Build history of the part. All positions in model axes, mm. Face numbers are marked on the shaded views. A direction names the side the tool comes from. Give positions to 0.01 mm unless a question says otherwise; leave off trailing zeros. Order: outer loops, then holes, each group sorted by start corner. A loop starts at its lowest first (then second) coordinate and runs counter-clockwise, first axis right, second up. Notation, with made-up numbers: M -8.5,77 L 15.5,77 A9 cw 15.5,93 Z; hole C 34.25,37.25 d7. An arc over 180 degrees is marked long. Use CSV: the item, a comma, the result in double quotes. Start each with the question number.
Item 1: Band-saw the part on A-A on y = 47.5. Write the cut outline in (x, z).
Item 2: Band-saw the part on B-B on z = 26. Write the cut outline in (x, y), plus the area to 3 significant figures.
Item 3: Wall check: line 1 along X through (y, z) = (41, 72); line 2 along Y through (x, z) = (24.5, 47.5); line 3 along X through (y, z) = (38, 25). Give the ranges that are in metal, low to high.
Item 4: Which spindle directions (+Z, -Z, +X, -X, +Y, -Y) get a long thin tool onto all of the face, cutting with end or side? Do the marked faces 1 and 2. Say none if no direction does.
Item 5: Band-saw the part on D-D on z = 61. Write the cut outline in (x, y), plus the area to 3 significant figures.
Item 6: Band-saw the part on C-C on x = 17.5. Write the cut outline in (y, z).
Item 7: Two-plate mould, pull along Z, no slides. Class the marked faces 3, 4 and 5: pulls with the +Z half, pulls with the -Z half, needs draft (parallel to the pull), parting line crosses it, or undercut.
Item 8: Pin check, flat tips, straight feed: P1, Ø13, axis at y = 42, z = 54.5, coming from the +X side; P2, Ø6, axis at y = 25, z = 65.5, coming from the +X side; P3, Ø8, axis at y = 18.5, z = 9.5, coming from the +X side; P4, Ø4, axis at x = -39.5, y = 34, coming from the -Z side. Stop position of each tip, or through.
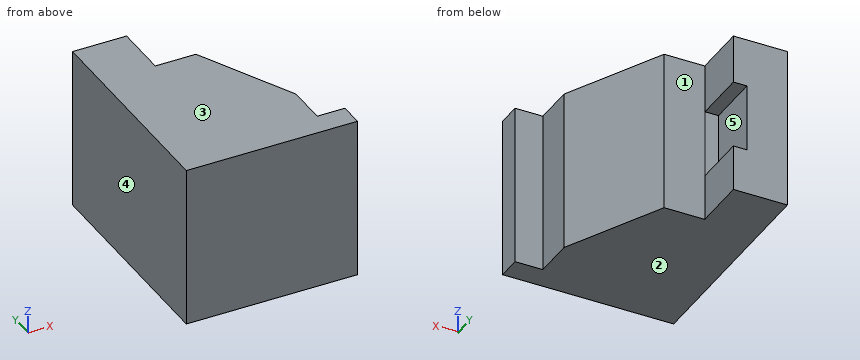
from build123d import *

# Parameters (mm, degrees)
F0_W      = 89.0809036791
F0_H      = 101.640611887
F1_DEPTH  = 76.2
F3_DEPTH  = 76.201
F4_R      = 10.6888946351
F3_FACE_W = 51.3844064591
F3_FACE_H = 76.2
F5_DEPTH  = 12.7
F8_W      = 6.35
F8_H      = 31.75
F9_DEPTH  = 25.4


# Not quite as in the source:
# - a feature of the source that left no trace in its solid (it failed there, or was rolled back) is left out


with BuildPart() as f1:
    # F0 (on Top) → F1 (new body)
    with BuildSketch(Plane.XY):
        with Locations((-6.628734991, 2.674754709)):
            Rectangle(F0_W, F0_H)
    extrude(amount=F1_DEPTH)

    # F2 (on face) → F3 (cut, through all)
    with BuildSketch(Plane.XY.offset(76.2)):
        Polygon((37.9117168486, 53.4950606525), (-25.8171800524, 53.4950606525), (-25.8171800524, 27.9104653746), (-6.7450297065, 27.9104653746), (16.0485189408, -18.1418024004), (16.0485189408, -36.9813665748), (29.0734022856, -36.9813665748), (29.0734022856, -48.1455512345), (31.1666838825, -48.1455512345), (37.9117168486, -48.1455512345), align=None)
    extrude(amount=-F3_DEPTH, mode=Mode.SUBTRACT)

    # F4 (on Right) + F3_face (on face) → F5 (join)
    with BuildSketch(Plane.YZ):
        with Locations((0, 59.542324394)):
            Circle(F4_R)
    with BuildSketch(Plane(origin=(4.6517446171, 4.8843314871, 38.1), x_dir=(-0.4435888282, 0.8962304121, 0), z_dir=(0.8962304121, 0.4435888282, 0))):
        Rectangle(F3_FACE_W, F3_FACE_H)
    extrude(amount=-F5_DEPTH, dir=(1, 0, 0))

    # F8 (on face) → F9 (cut)
    with BuildSketch(Plane(origin=(0, 53.4950606525, 0), x_dir=(-1, 0, 0), z_dir=(0, 1, 0))):
        with Locations((28.9921800524, 37.465)):
            Rectangle(F8_W, F8_H)
    extrude(amount=-F9_DEPTH, mode=Mode.SUBTRACT)


solid = f1.part
Model answer:
1,outline,"M -51.17,0 L -25.82,0 L -25.82,21.59 L -32.17,21.59 L -32.17,53.34 L -25.82,53.34 L -25.82,76.2 L -51.17,76.2 Z"
2,outline,"M -51.17,-48.15 L 29.07,-48.15 L 29.07,-36.98 L 16.05,-36.98 L 16.05,-18.14 L -6.75,27.91 L -25.82,27.91 L -25.82,28.1 L -32.17,28.1 L -32.17,53.5 L -51.17,53.5 Z"
2,area,"5,220 mm^2"
3,line 1,"x = -51.17 to -25.82"
3,line 2,"y = -48.15 to -36.98"
3,line 3,"x = -51.17 to -32.17"
4,face 1,"+Z, -Z, +X, +Y"
4,face 2,"-Z, +X, -X, +Y, -Y"
5,outline,"M -51.17,-48.15 L 29.07,-48.15 L 29.07,-36.98 L 16.05,-36.98 L 16.05,-18.14 L -6.75,27.91 L -25.82,27.91 L -25.82,53.5 L -51.17,53.5 Z"
5,area,"5,380 mm^2"
6,outline,"M -48.15,0 L -36.98,0 L -36.98,76.2 L -48.15,76.2 Z"
7,face 3,"pulls with the +Z half"
7,face 4,"needs draft"
7,face 5,"undercut"
8,P1,"stops at x = -25.82"
8,P2,"stops at x = -3.82"
8,P3,"stops at x = -0.11"
8,P4,"stops at z = 0"
